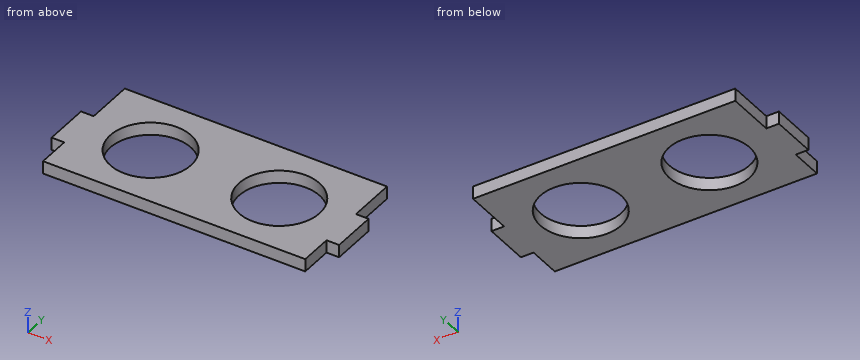
Autodesk Fusion 360 part; units mm, degrees
sketch "Sketch1" plane through (0, 0, 0) normal (0, 0, 1) x (1, 0, 0)
  line L0 (15, 60) -> (67, 60)
  line L1 (67, 60) -> (67, 50.5)
  line L2 (15, 60) -> (15, 50.5)
  line L3 (67, 50.5) -> (69.5, 50.5)
  line L4 (15, 50.5) -> (12.5, 50.5)
  line L5 (69.5, 50.5) -> (69.5, 41.5)
  line L6 (12.5, 50.5) -> (12.5, 41.5)
  line L7 (69.5, 41.5) -> (67, 41.5)
  line L8 (12.5, 41.5) -> (15, 41.5)
  line L9 (67, 41.5) -> (67, 35)
  line L10 (15, 41.5) -> (15, 35)
  line L11 (67, 35) -> (15, 35)
  line L12 (15, 35) -> (15, 29) construction
  circle A0 centre (28.3, 47.4) radius 8
  line L13 (28.3, 47.4) -> (53.8, 47.4) construction
  circle A1 centre (53.8, 47.4) radius 8
  dimension "d1" = 52
  dimension "d2" = 9.5
  dimension "d3" = 9.5
  dimension "d4" = 2.5
  dimension "d5" = 2.5
  dimension "d6" = 9
  dimension "d7" = 9
  dimension "d8" = 2.5
  dimension "d9" = 2.5
  dimension "d10" = 6.5
  dimension "d11" = 6.5
  dimension "d12" = 16
  dimension "d13" = 12.4
  dimension "d14" = 15.8
  dimension "d15" = 25.5
  dimension "d16" = 16
extrude "Extrude1" add sketch "Sketch1" along normal blind 2.5
The listing builds one solid part. Answer for the finished solid, in the listing's coordinates (mm). Round coordinates to 2 decimals unless told otherwise and drop trailing zeros. Loops run counter-clockwise (first coordinate to the right, second up) from the corner with the lowest first, then second, coordinate; pieces in that order, holes last.
1) Consider line 1 (X direction, y = 47.25, z = 2.2); line 2 (Y direction, x = 53.8, z = 1.55); line 3 (X direction, y = 54, z = 1.75). Determine where each line is inside the solid, lowest interval first.
Outcome:
line 1: x = 12.5 to 20.3, 36.3 to 45.8, 61.8 to 69.5
line 2: y = 35 to 39.4, 55.4 to 60
line 3: x = 15 to 23.78, 32.82 to 49.28, 58.32 to 67
2) A cutting plane is placed at C-C on y = 47.4. Determine the outline of the cut face in (x, z), plus the area to 3 significant figures.
Outcome:
outline: (12.5, 0) - (20.3, 0) - (20.3, 2.5) - (12.5, 2.5) - close; (36.3, 0) - (45.8, 0) - (45.8, 2.5) - (36.3, 2.5) - close; (61.8, 0) - (69.5, 0) - (69.5, 2.5) - (61.8, 2.5) - close
area: 62.5 mm2
3) Given P1, Ø2, axis at x = 25, y = 42, coming from the +Z side; P2, Ø0.8, axis at y = 38, z = 1, coming from the +X side; P3, Ø0.8, axis at x = 68.5, z = 1.5, coming from the -Y side; P4, Ø10, axis at x = 51, y = 46, coming from the -Z side, each flat-ended and moving along its own axis, determine where each tip first touches the part or whether it passes through.
Outcome:
P1: passes through
P2: stops at x = 67
P3: stops at y = 41.5
P4: stops at z = 0
4) A cutting plane is placed at A-A on x = 53.8. Determine the outline of the cut face in (y, z), plus the area to 3 significant figures.
Outcome:
outline: (35, 0) - (39.4, 0) - (39.4, 2.5) - (35, 2.5) - close; (55.4, 0) - (60, 0) - (60, 2.5) - (55.4, 2.5) - close
area: 22.5 mm2
5) A cutting plane is placed at D-D on x = 28. Determine the outline of the cut face in (y, z).
Outcome:
outline: (35, 0) - (39.41, 0) - (39.41, 2.5) - (35, 2.5) - close; (55.39, 0) - (60, 0) - (60, 2.5) - (55.39, 2.5) - close
6) A cutting plane is placed at B-B on z = 1.65. Determine the outline of the cut face in (x, y).
Outcome:
outline: (12.5, 41.5) - (15, 41.5) - (15, 35) - (67, 35) - (67, 41.5) - (69.5, 41.5) - (69.5, 50.5) - (67, 50.5) - (67, 60) - (15, 60) - (15, 50.5) - (12.5, 50.5) - close; hole circle Ø16 at (28.3, 47.4); hole circle Ø16 at (53.8, 47.4)
